Source: CAD feature listing. Evaluate the final solid. Frame: model axes, mm. Face numbers are marked on the shaded views. A direction names the side the tool comes from. Coordinates: 2 decimals unless noted, no trailing zeros. Write each loop counter-clockwise with the first axis right and the second up, starting at its lowest first coordinate (ties: lowest second). Pieces come first, ordered by that corner, then holes. Notation, with made-up numbers: (54.25, -29.75) - (58.25, -29.75) arc R25 ccw to (58.25, 8.25) - close; hole circle Ø3 at (-17.5, 80.25). An arc over 180 degrees is marked (long way). One line per item, written item: value.
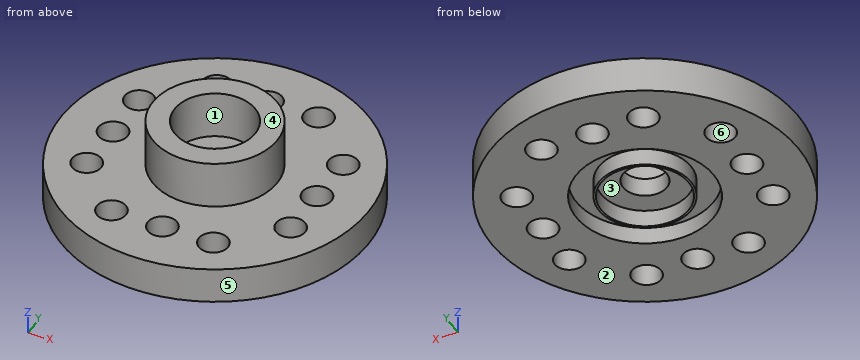
from build123d import *

# Parameters (mm, degrees)
SKETCH1_R           = 10.5
BOSS_EXTRUDE1_DEPTH = 2.5
SKETCH2_R           = 4.25
SKETCH2_R_2         = 2.75
BOSS_EXTRUDE2_DEPTH = 3.3
SKETCH3_R           = 1.5
CUT_EXTRUDE1_DEPTH  = 16.941769036
SKETCH3_3_R         = 4.7
SKETCH3_3_R_2       = 1.5
CUT_EXTRUDE2_DEPTH  = 1.2
SKETCH4_R           = 3.15
SKETCH4_R_2         = 3
BOSS_EXTRUDE3_DEPTH = 1.2
SKETCH5_R           = 1
CUT_EXTRUDE3_DEPTH  = 16.941769036


with BuildPart() as part:
    # Sketch1 → Boss-Extrude1 (new body)
    with BuildSketch(Plane.XY):
        Circle(SKETCH1_R)
    extrude(amount=BOSS_EXTRUDE1_DEPTH)

    # Sketch2 → Boss-Extrude2 (add)
    with BuildSketch(Plane.XY.offset(2.5)):
        Circle(SKETCH2_R)
        Circle(SKETCH2_R_2, mode=Mode.SUBTRACT)
    extrude(amount=BOSS_EXTRUDE2_DEPTH)

    # Sketch3 → Cut-Extrude1 (cut, through all)
    with BuildSketch(Plane(origin=(0, 0, 0), x_dir=(-1, 0, 0), z_dir=(0, 0, -1))):
        Circle(SKETCH3_R)
    extrude(amount=-CUT_EXTRUDE1_DEPTH, mode=Mode.SUBTRACT)

    # Sketch3<3> → Cut-Extrude2 (cut)
    with BuildSketch(Plane(origin=(0, 0, 0), x_dir=(-1, 0, 0), z_dir=(0, 0, -1))):
        Circle(SKETCH3_3_R)
        Circle(SKETCH3_3_R_2, mode=Mode.SUBTRACT)
    extrude(amount=-CUT_EXTRUDE2_DEPTH, mode=Mode.SUBTRACT)

    # Sketch4 → Boss-Extrude3 (add)
    with BuildSketch(Plane(origin=(0, 0, 1.2), x_dir=(-1, 0, 0), z_dir=(0, 0, -1))):
        Circle(SKETCH4_R)
        Circle(SKETCH4_R_2, mode=Mode.SUBTRACT)
    extrude(amount=BOSS_EXTRUDE3_DEPTH)

    # Sketch5 → Cut-Extrude3 (cut, through all)
    with BuildSketch(Plane(origin=(0, 0, 0), x_dir=(-1, 0, 0), z_dir=(0, 0, -1))):
        with Locations((0, 7)):
            Circle(SKETCH5_R)
        with Locations((0, -7)):
            Circle(SKETCH5_R)
        with Locations((-7, 0)):
            Circle(SKETCH5_R)
        with Locations((7, 0)):
            Circle(SKETCH5_R)
        with Locations((3.5, 7)):
            Circle(SKETCH5_R)
        with Locations((-3.5, 7)):
            Circle(SKETCH5_R)
        with Locations((-7, 3.5)):
            Circle(SKETCH5_R)
        with Locations((-7, -3.5)):
            Circle(SKETCH5_R)
        with Locations((7, -3.5)):
            Circle(SKETCH5_R)
        with Locations((7, 3.5)):
            Circle(SKETCH5_R)
        with Locations((-3.5, -7)):
            Circle(SKETCH5_R)
        with Locations((3.5, -7)):
            Circle(SKETCH5_R)
    extrude(amount=-CUT_EXTRUDE3_DEPTH, mode=Mode.SUBTRACT)


solid = part.part
1) Section query C-C on y = -3.5. Output: boundary loops of the cut face in (x, z).
Values found:
outline: (-9.9, 0) - (-8, 0) - (-8, 2.5) - (-9.9, 2.5) - close; (-6, 0) - (-3.14, 0) - (-3.14, 1.2) - (3.14, 1.2) - (3.14, 0) - (6, 0) - (6, 2.5) - (2.41, 2.5) - (2.41, 5.8) - (-2.41, 5.8) - (-2.41, 2.5) - (-6, 2.5) - close; (8, 0) - (9.9, 0) - (9.9, 2.5) - (8, 2.5) - close
2) Material intervals for line 1 (Y direction, x = 0, z = 1.6); line 2 (Y direction, x = -7, z = 1.35); line 3 (Y direction, x = -4.25, z = 1.7), sorted ascending.
Values found:
line 1: -10.5 to -8, -6 to -1.5, 1.5 to 6, 8 to 10.5
line 2: -7.83 to -4.5, -2.5 to -1, 1 to 2.5, 4.5 to 7.83
line 3: -9.6 to -7.66, -6.34 to 6.34, 7.66 to 9.6
3) Section query B-B on x = -6.75. Output: boundary loops of the cut face in (y, z).
Values found:
outline: (-8.04, 0) - (-4.47, 0) - (-4.47, 2.5) - (-8.04, 2.5) - close; (-2.53, 0) - (-0.97, 0) - (-0.97, 2.5) - (-2.53, 2.5) - close; (0.97, 0) - (2.53, 0) - (2.53, 2.5) - (0.97, 2.5) - close; (4.47, 0) - (8.04, 0) - (8.04, 2.5) - (4.47, 2.5) - close
4) Reachability of the marked faces 1, 2 and 3 from +Z, -Z, +X, -X, +Y, -Y: full face, straight path, thin tool, end or side. Return the list, or none.
Values found:
face 1: +Z
face 2: -Z, +X, -X, +Y, -Y
face 3: -Z
5) Draft query along X for the marked faces 4, 5 and 6. Return one class per face: released by +X, released by -X, zero draft, split by the parting line, or undercut.
Values found:
face 4: zero draft
face 5: split by the parting line
face 6: undercut
6) Section query A-A on z = 0.5. State how many separate pieces and enclosed holes the cut face has, then the cut area to 3 significant figures.
Values found:
separate pieces: 2
enclosed holes: 14
area: 242 mm2
7) Contact query for a flat-ended pin moving along its axis: P1, Ø2.5, axis at x = -3.5, y = 7, coming from the +Z side. Output: stop coordinate, or through.
Values found:
P1: z = 2.5
